Here's the drawing with two shaded views (mm, measured from the low corner). I have some questions. Give positions to 0.01 mm unless a question says otherwise; leave off trailing zeros. Loops run counter-clockwise (first coordinate to the right, second up) from the corner with the lowest first, then second, coordinate; pieces in that order, holes last. Notation, with made-up numbers: M 0,40.5 L 7,40.5 A14 ccw 7,66.5 Z; hole C 68,0.25 d9. An arc over 180 degrees is marked long. Put each result on its own line as item: value. Start each with the question number.
1) Imagine slicing it at A-A (x = 77.5). Write out the boundary of the cut face in (y, z) (1 decimal).
2) Imagine slicing it at D-D (y = 71.5). Write out the boundary of the cut face in (x, z), then the cut area to 3 significant figures.
3) For P1, Ø1.5, axis at y = 121.5, z = 2, coming from the -X side; P2, Ø1.5, axis at y = 24.5, z = 2, coming from the +X side; P3, Ø0.9, axis at x = 110, z = 1, coming from the +Y side; P4, Ø1.5, axis at x = 32.5, y = 16, coming from the -Z side, each with a flat end and sliding along its axis, tell me the tip position at first contact or that it passes through.
4) Imagine slicing it at B-B (y = 132). Write out the boundary of the cut face in (x, z) (1 decimal).
5) Please list where these lines run through material, in increasing order: line 1 along Y through (x, z) = (79.5, 0.7) (1 decimal); line 2 along X through (y, z) = (25.5, 0.25) (1 decimal); line 3 along X through (y, z) = (26.5, 0.45) (1 decimal). Write a range as from..to.
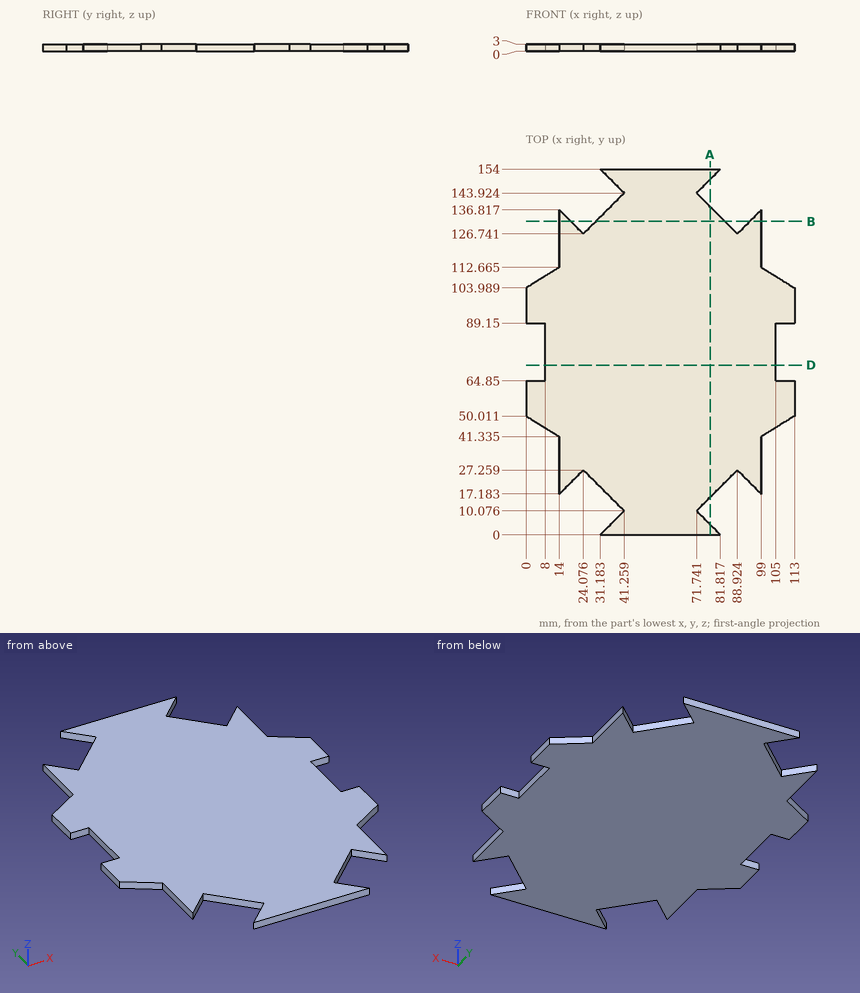
Recorded:
1. outline: M 0,0 L 4.3,0 L 4.3,3 L 0,3 Z; M 15.8,0 L 138.2,0 L 138.2,3 L 15.8,3 Z; M 149.7,0 L 154,0 L 154,3 L 149.7,3 Z
2. outline: M 8,0 L 105,0 L 105,3 L 8,3 Z
2. area: 291 mm²
3. P1: x = 14
3. P2: x = 99
3. P3: y = 106.13
3. P4: through
4. outline: M 14,0 L 18.8,0 L 18.8,3 L 14,3 Z; M 29.3,0 L 83.7,0 L 83.7,3 L 29.3,3 Z; M 94.2,0 L 99,0 L 99,3 L 94.2,3 Z
5. line 1: 0..2.3, 17.8..136.2, 151.7..154
5. line 2: 14..22.3, 25.8..87.2, 90.7..99
5. line 3: 14..23.3, 24.8..88.2, 89.7..99
